```python
from build123d import *

# Parameters (mm, degrees)
SKETCH1_R           = 1.5
BOSS_EXTRUDE1_DEPTH = 4
SKETCH2_R           = 1.5
CUT_EXTRUDE1_DEPTH  = 10


with BuildPart() as part:
    # Sketch1 → Boss-Extrude1 (new body)
    with BuildSketch(Plane(origin=(0, 0, 0), x_dir=(1, 0, 0), z_dir=(0, 1, 0))):
        with BuildLine():
            Line((-48.071067812, 30), (-48.071067812, -30))
            Line((-48.071067812, -30), (-41.535533906, -36.535533906))
            ThreePointArc((-41.535533906, -36.535533906), (-39.913417162, -37.619397663), (-38, -38))
            Line((-38, -38), (38, -38))
            ThreePointArc((38, -38), (39.913417162, -37.619397663), (41.535533906, -36.535533906))
            Line((41.535533906, -36.535533906), (48.071067812, -30))
            Line((48.071067812, -30), (48.071067812, 30))
            Line((48.071067812, 30), (41.535533906, 36.535533906))
            ThreePointArc((41.535533906, 36.535533906), (39.913417162, 37.619397663), (38, 38))
            Line((38, 38), (-38, 38))
            ThreePointArc((-38, 38), (-39.913417162, 37.619397663), (-41.535533906, 36.535533906))
            Line((-41.535533906, 36.535533906), (-48.071067812, 30))
        make_face()
        with Locations(Location((32.059596398, -28.691611003, 0), (0, 0, 270))):
            Circle(SKETCH1_R, mode=Mode.SUBTRACT)
        with Locations(Location((32.059596398, 28.458388997, 0), (0, 0, 270))):
            Circle(SKETCH1_R, mode=Mode.SUBTRACT)
        with Locations(Location((-31.440403602, -28.691611003, 0), (0, 0, 270))):
            Circle(SKETCH1_R, mode=Mode.SUBTRACT)
        with Locations(Location((-31.440403602, 28.458388997, 0), (0, 0, 270))):
            Circle(SKETCH1_R, mode=Mode.SUBTRACT)
        with BuildLine():
            Line((26.770818028, 21.768665175), (26.783167828, 24.768639755))
            ThreePointArc((26.783167828, 24.768639755), (26.493187967, 25.476946269), (25.787292902, 25.772747882))
            Line((25.787292902, 25.772747882), (12.787403054, 25.826263684))
            ThreePointArc((12.787403054, 25.826263684), (12.07909654, 25.536283823), (11.783294927, 24.830388757))
            Line((11.783294927, 24.830388757), (11.770945126, 21.830414177))
            ThreePointArc((11.770945126, 21.830414177), (12.060924988, 21.122107663), (12.766820053, 20.82630605))
            Line((12.766820053, 20.82630605), (25.766709901, 20.772790248))
            ThreePointArc((25.766709901, 20.772790248), (26.475016415, 21.062770109), (26.770818028, 21.768665175))
        make_face(mode=Mode.SUBTRACT)
        with BuildLine():
            Line((28.613064126, -11.166765747), (28.613064126, 10.833234253))
            ThreePointArc((28.613064126, 10.833234253), (28.173724298, 11.893894425), (27.113064126, 12.333234253))
            Line((27.113064126, 12.333234253), (22.113064126, 12.333234253))
            ThreePointArc((22.113064126, 12.333234253), (21.052403954, 11.893894425), (20.613064126, 10.833234253))
            Line((20.613064126, 10.833234253), (20.613064126, -11.166765747))
            ThreePointArc((20.613064126, -11.166765747), (21.052403954, -12.227425919), (22.113064126, -12.666765747))
            Line((22.113064126, -12.666765747), (27.113064126, -12.666765747))
            ThreePointArc((27.113064126, -12.666765747), (28.173724298, -12.227425919), (28.613064126, -11.166765747))
        make_face(mode=Mode.SUBTRACT)
        with BuildLine():
            Line((26.680500347, -25.110893415), (26.680500347, -22.110893415))
            ThreePointArc((26.680500347, -22.110893415), (26.387607128, -21.403786634), (25.680500347, -21.110893415))
            Line((25.680500347, -21.110893415), (12.680500347, -21.110893415))
            ThreePointArc((12.680500347, -21.110893415), (11.973393565, -21.403786634), (11.680500347, -22.110893415))
            Line((11.680500347, -22.110893415), (11.680500347, -25.110893415))
            ThreePointArc((11.680500347, -25.110893415), (11.973393565, -25.818000196), (12.680500347, -26.110893415))
            Line((12.680500347, -26.110893415), (25.680500347, -26.110893415))
            ThreePointArc((25.680500347, -26.110893415), (26.387607128, -25.818000196), (26.680500347, -25.110893415))
        make_face(mode=Mode.SUBTRACT)
        with BuildLine():
            Line((-37.071067812, 15.952856913), (-19.071067812, 15.952856913))
            ThreePointArc((-19.071067812, 15.952856913), (-18.363961031, 15.659963694), (-18.071067812, 14.952856913))
            Line((-18.071067812, 14.952856913), (-18.071067812, 13.952856913))
            ThreePointArc((-18.071067812, 13.952856913), (-18.363961031, 13.245750131), (-19.071067812, 12.952856913))
            Line((-19.071067812, 12.952856913), (-37.071067812, 12.952856913))
            ThreePointArc((-37.071067812, 12.952856913), (-37.778174593, 13.245750131), (-38.071067812, 13.952856913))
            Line((-38.071067812, 13.952856913), (-38.071067812, 14.952856913))
            ThreePointArc((-38.071067812, 14.952856913), (-37.778174593, 15.659963694), (-37.071067812, 15.952856913))
        make_face(mode=Mode.SUBTRACT)
        with BuildLine():
            Line((6.394530071, 14.952856913), (6.394530071, 13.952856913))
            ThreePointArc((6.394530071, 13.952856913), (6.101636852, 13.245750131), (5.394530071, 12.952856913))
            Line((5.394530071, 12.952856913), (-12.605469929, 12.952856913))
            ThreePointArc((-12.605469929, 12.952856913), (-13.312576711, 13.245750131), (-13.605469929, 13.952856913))
            Line((-13.605469929, 13.952856913), (-13.605469929, 14.952856913))
            ThreePointArc((-13.605469929, 14.952856913), (-13.312576711, 15.659963694), (-12.605469929, 15.952856913))
            Line((-12.605469929, 15.952856913), (5.394530071, 15.952856913))
            ThreePointArc((5.394530071, 15.952856913), (6.101636852, 15.659963694), (6.394530071, 14.952856913))
        make_face(mode=Mode.SUBTRACT)
        with BuildLine():
            Line((-38.071067812, -14.952856913), (-38.071067812, -13.952856913))
            ThreePointArc((-38.071067812, -13.952856913), (-37.778174593, -13.245750131), (-37.071067812, -12.952856913))
            Line((-37.071067812, -12.952856913), (-19.071067812, -12.952856913))
            ThreePointArc((-19.071067812, -12.952856913), (-18.363961031, -13.245750131), (-18.071067812, -13.952856913))
            Line((-18.071067812, -13.952856913), (-18.071067812, -14.952856913))
            ThreePointArc((-18.071067812, -14.952856913), (-18.363961031, -15.659963694), (-19.071067812, -15.952856913))
            Line((-19.071067812, -15.952856913), (-37.071067812, -15.952856913))
            ThreePointArc((-37.071067812, -15.952856913), (-37.778174593, -15.659963694), (-38.071067812, -14.952856913))
        make_face(mode=Mode.SUBTRACT)
        with BuildLine():
            Line((-13.605469929, -14.952856913), (-13.605469929, -13.952856913))
            ThreePointArc((-13.605469929, -13.952856913), (-13.312576711, -13.245750131), (-12.605469929, -12.952856913))
            Line((-12.605469929, -12.952856913), (5.394530071, -12.952856913))
            ThreePointArc((5.394530071, -12.952856913), (6.101636852, -13.245750131), (6.394530071, -13.952856913))
            Line((6.394530071, -13.952856913), (6.394530071, -14.952856913))
            ThreePointArc((6.394530071, -14.952856913), (6.101636852, -15.659963694), (5.394530071, -15.952856913))
            Line((5.394530071, -15.952856913), (-12.605469929, -15.952856913))
            ThreePointArc((-12.605469929, -15.952856913), (-13.312576711, -15.659963694), (-13.605469929, -14.952856913))
        make_face(mode=Mode.SUBTRACT)
    extrude(amount=BOSS_EXTRUDE1_DEPTH)

    # Sketch2 → Cut-Extrude1 (cut)
    with BuildSketch(Plane(origin=(0, 4, 0), x_dir=(1, 0, 0), z_dir=(0, 1, 0))):
        with Locations(Location((-40.071067812, 30, 0), (0, 0, 270))):
            Circle(SKETCH2_R)
        with Locations(Location((40.071067812, 30, 0), (0, 0, 270))):
            Circle(SKETCH2_R)
        with Locations(Location((40.071067812, -30, 0), (0, 0, 270))):
            Circle(SKETCH2_R)
        with Locations(Location((-40.071067812, -30, 0), (0, 0, 270))):
            Circle(SKETCH2_R)
    extrude(amount=-CUT_EXTRUDE1_DEPTH, mode=Mode.SUBTRACT)


solid = part.part
```
Check sheet for the modelled part. Datum: model origin and axes. Units: mm. A direction names the side the tool comes from. Give positions to 0.01 mm unless a question says otherwise; leave off trailing zeros. Order: outer loops, then holes, each group sorted by start corner. A loop starts at its lowest first (then second) coordinate and runs counter-clockwise, first axis right, second up. Notation, with made-up numbers: M 74.5,17.5 L 119.5,17.5 A10 ccw 119.5,30.5 Z; hole C 51.5,15 d6. An arc over 180 degrees is marked long. Answer in a Markdown table with one row per item.
1) Access from +Z, -Z, +X, -X, +Y, -Y to the whole of each face (thin tool, end or side, straight path). Record for faces 4 (the flat face through (25, 2, 12.667)), 5 (the cylindrical face through (-39.89, 1.97, -37.63)).
Filled sheet:
| item | result |
|---|---|
| face 4 | +Y, -Y |
| face 5 | -Z, -X, +Y, -Y |
2) Cross-section at A-A, the plane z = 5. Enter the section's corners in (x, y), plus the area to 3 significant figures.
Filled sheet:
| item | result |
|---|---|
| outline | M -48.07,0 L 20.61,0 L 20.61,4 L -48.07,4 Z; M 28.61,0 L 48.07,0 L 48.07,4 L 28.61,4 Z |
| area | 353 mm2 |
3) Cross-section at D-D, the plane z = -23. Enter the section's corners in (x, y), plus the area to 3 significant figures.
Filled sheet:
| item | result |
|---|---|
| outline | M -48.07,0 L 11.78,0 L 11.78,4 L -48.07,4 Z; M 26.78,0 L 48.07,0 L 48.07,4 L 26.78,4 Z |
| area | 325 mm2 |
4) Gauge pin test, flat end, axial feed: P1, Ø2.5, axis at x = 40.07, z = 30, coming from the +Y side. Record the tip position at first contact, or that the pin passes through.
Filled sheet:
| item | result |
|---|---|
| P1 | passes through |
5) Cross-section at C-C, the plane y = 0.65. Count the separate pieces of the cut face and the enclosed holes in it, plus the area to 3 significant figures.
Filled sheet:
| item | result |
|---|---|
| separate pieces | 1 |
| enclosed holes | 15 |
| area | 6,540 mm2 |
6) Cross-section at B-B, the plane x = -24.5. Enter the section's corners in (y, z), plus the area to 3 significant figures.
Filled sheet:
| item | result |
|---|---|
| outline | M 0,-38 L 4,-38 L 4,-15.95 L 0,-15.95 Z; M 0,-12.95 L 4,-12.95 L 4,12.95 L 0,12.95 Z; M 0,15.95 L 4,15.95 L 4,38 L 0,38 Z |
| area | 280 mm2 |
7) Release check for a two-part mould opening along Z. For faces 1 (the cylindrical face through (-39.94, 1.97, 37.61)), 2 (the cylindrical face through (39.94, 1.97, -37.61)), 3 (the cylindrical face through (-40, 2, -31.5)) record: +Z half, -Z half, draft (parallel to the pull), parting line (faces both ways), or undercut.
Filled sheet:
| item | result |
|---|---|
| face 1 | +Z half |
| face 2 | -Z half |
| face 3 | undercut |
8) Thickness scan on L1, parallel to Z at x = 1.5, y = 2.8; L2, parallel to Z at x = 17, y = 1.5; L3, parallel to X at y = 1.8, z = -27.5. Record the ranges inside material, lowest first. Write a range as [from, to].
Filled sheet:
| item | result |
|---|---|
| L1 | z = [-38, -15.95], [-12.95, 12.95], [15.95, 38] |
| L2 | z = [-38, -25.81], [-20.81, 21.11], [26.11, 38] |
| L3 | x = [-48.07, -32.59], [-30.29, 30.91], [33.21, 48.07] |
